Read the model definition and answer for the solid it produces. Units are mm, in the model's axes. Face numbers are marked on the shaded views. Coordinates: 2 decimals unless noted, no trailing zeros. Loops run counter-clockwise (first coordinate to the right, second up) from the corner with the lowest first, then second, coordinate; pieces in that order, holes last. Notation, with made-up numbers: (-8.5, 27) -> (14.5, 27) arc R8 cw to (14.5, 36) -> close; hole circle Ø3 at (-15, -16). An arc over 180 degrees is marked (long way). Answer as a JSON object with one key per item and string values. Group by question number.
1) Section C-C, the plane x = 12 is taken. Give the vertices of the cut face in (y, z), plus the area to 3 significant figures.
2) Determine the mould class of the marked faces 1, 2 and 3 for opening direction Z: released by +Z, released by -Z, zero draft, split by the parting line, or undercut.
3) Section B-B, the plane z = -2.5 is taken. Count the separate pieces of the cut face and the enclosed holes in it, plus the area to 3 significant figures.
4) Flat-ended cylindrical pins translate along their axes: P1, Ø3, axis at x = 2, y = -11, coming from the -Z side; P2, Ø10, axis at y = -11, z = -28.5, coming from the +X side. Find the tip coordinate at first contact, or state that the pin passes through.
5) Consider probe 1 along Z at (x, y) = (11.5, -23.75); probe 2 along Z at (x, y) = (17, -1.5). Determine where each line is inside the solid, lowest interval first. Write a range as [from, to].
6) Section A-A, the plane z = -17.5 is taken. Give the vertices of the cut face in (x, y).
7) Section D-D, the plane y = -5.75 is taken. Give the vertices of the cut face in (x, z), plus the area to 3 significant figures.
from build123d import *

# Parameters (mm, degrees)
F1_DEPTH = 27.5
F3_DEPTH = 32.001
F4_R     = 1
F6_DEPTH = 26.001


# Not quite as in the source:
# - ends of sketch curves that miss each other by under 0.0002 mm in the source are joined
# - a feature names something its author has since deleted; it is built from what else it names


with BuildPart() as f1:
    # F0 (on Right) → F1 (new body, symmetric)
    with BuildSketch(Plane.YZ):
        Polygon((0, -32), (0, 0), (-26, 0), (-26, -4), (-4, -4), (-4, -32), align=None)
    extrude(amount=F1_DEPTH, both=True)

    # F2 (on Top) → F3 (cut, through all)
    with BuildSketch(Plane.XY):
        with BuildLine():
            Line((-17.55, -21), (-20.95, -21))
            ThreePointArc((-20.95, -21), (-19.25, -22.7), (-17.55, -21))
        make_face()
        with BuildLine():
            Line((-20.95, -12.6989117458), (-20.95, -21))
            Line((-20.95, -21), (-17.55, -21))
            Line((-17.55, -21), (-17.55, -12.6989117458))
            Line((-17.55, -12.6989117458), (-17.55, -12.6936758503))
            ThreePointArc((-17.55, -12.6936758503), (-19.2526179384, -10.9989137616), (-20.95, -12.6989117458))
        make_face()
        with BuildLine():
            ThreePointArc((17.55, -21), (19.25, -22.7), (20.95, -21))
            Line((20.95, -21), (17.55, -21))
        make_face()
        with BuildLine():
            Line((17.55, -21), (20.95, -21))
            Line((20.95, -21), (20.95, -12.6989117458))
            ThreePointArc((20.95, -12.6989117458), (19.2526179384, -10.9989137616), (17.5500080631, -12.6936758752))
            ThreePointArc((17.5500080631, -12.6936758752), (17.5500020158, -12.6962938074), (17.55, -12.6989117458))
            Line((17.55, -12.6989117458), (17.55, -21))
        make_face()
    extrude(amount=-F3_DEPTH, mode=Mode.SUBTRACT)

    # F4
    f4_edges = [f1.edges().sort_by_distance(p)[0] for p in [
        (0, 0, -32),
        (-27.5, 0, -16),
        (27.5, 0, -16),
        (0, 0, 0),
        (0, -26, 0),
        (-27.5, -13, 0),
        (27.5, -13, 0),
    ]]
    fillet(f4_edges, radius=F4_R)

    # F5 (on face) → F6 (cut, through all)
    with BuildSketch(Plane(origin=(0, 0, 0), x_dir=(-1, 0, 0), z_dir=(0, 1, 0))):
        with BuildLine():
            Line((15.85, -11.7517232777), (15.85, -21.7517232777))
            ThreePointArc((15.85, -21.7517232777), (17.5, -23.4017232777), (19.15, -21.7517232777))
            Line((19.15, -21.7517232777), (19.15, -11.7517232777))
            ThreePointArc((19.15, -11.7517232777), (17.5, -10.1017232777), (15.85, -11.7517232777))
        make_face()
        with BuildLine():
            ThreePointArc((-19.15, -21.7517232777), (-17.5, -23.4017232777), (-15.85, -21.7517232777))
            Line((-15.85, -21.7517232777), (-15.85, -11.7517232777))
            ThreePointArc((-15.85, -11.7517232777), (-17.5, -10.1017232777), (-19.15, -11.7517232777))
            Line((-19.15, -11.7517232777), (-19.15, -21.7517232777))
        make_face()
    extrude(amount=-F6_DEPTH, mode=Mode.SUBTRACT)


solid = f1.part
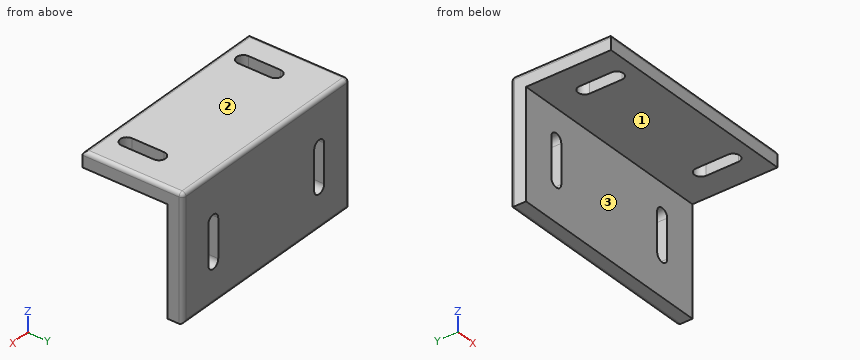
Determined:
{
 "1": {"outline": "(-26, -4) -> (-4, -4) -> (-4, -32) -> (-1, -32) arc R1 ccw to (0, -31) -> (0, -1) arc R1 ccw to (-1, 0) -> (-25, 0) arc R1 ccw to (-26, -1) -> close", "area": "215 mm²"},
 "2": {"face 1": "released by -Z", "face 2": "released by +Z", "face 3": "zero draft"},
 "3": {"separate pieces": "1", "enclosed holes": "2", "area": "1,350 mm²"},
 "4": {"P1": "z = -4", "P2": "through"},
 "5": {"probe 1": "[-4, 0]", "probe 2": "[-32, -23.32], [-10.18, 0]"},
 "6": {"outline": "(-27.5, -4) -> (-19.15, -4) -> (-19.15, 0) -> (-26.5, 0) arc R1 ccw to (-27.5, -1) -> close; (-15.85, -4) -> (15.85, -4) -> (15.85, 0) -> (-15.85, 0) -> close; (19.15, -4) -> (27.5, -4) -> (27.5, -1) arc R1 ccw to (26.5, 0) -> (19.15, 0) -> close"},
 "7": {"outline": "(-27.5, -4) -> (27.5, -4) -> (27.5, -1) arc R1 ccw to (26.5, 0) -> (-26.5, 0) arc R1 ccw to (-27.5, -1) -> close", "area": "220 mm²"}
}
